Geometry: final body of the model. Coordinates: model frame, mm. Give positions to 0.01 mm unless a question says otherwise; leave off trailing zeros. Order: outer loops, then holes, each group sorted by start corner. A loop starts at its lowest first (then second) coordinate and runs counter-clockwise, first axis right, second up. Notation, with made-up numbers: (33.25, 43.25) -> (41.25, 43.25) arc R29 ccw to (41.25, 81.25) -> close; hole circle Ø4 at (74, 11). An arc over 180 degrees is marked (long way). Answer in a Markdown table with one row per item. Add a question column.
Q1. Contact query for flat-ended pins moving along their axis: P1, Ø0.7, axis at x = -114, z = 0.5, coming from the +Y side; P2, Ø0.7, axis at y = 174.5, z = 0.5, coming from the +X side. Output: stop coordinate, or through.
Q2. Cut plane C-C on y = 148.5. Return the cut outline in (x, z).
Q3. Cut plane B-B on x = -333.5. Return the cut outline in (y, z), and give its area (3 significant figures).
Q4. Cut plane A-A on z = 0.8. Return the cut outline in (x, y).
Q5. Line query: line 1 along Y through (x, z) = (-56, 0.35); line 2 along X through (y, z) = (202, 1.15). Output: solid intervals per line, ascending. Write a range as from..to.
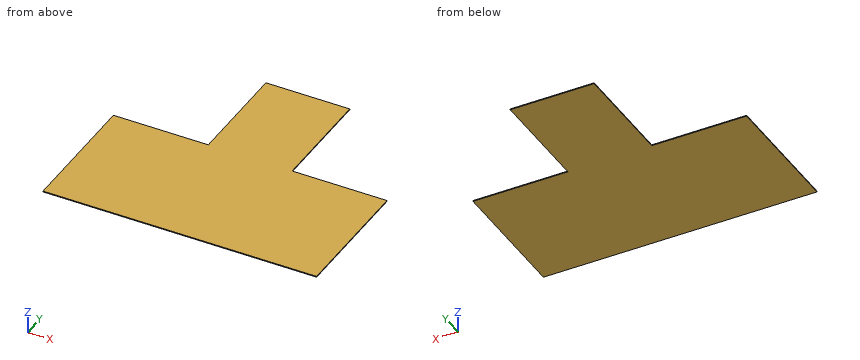
from build123d import *

# Parameters (mm, degrees)
F1_DEPTH = 1.4111111111
F2_DEPTH = 101.2317
F3_DEPTH = 66.675
F4_DEPTH = 66.675
F5_DEPTH = 47.498


# Not quite as in the source:
# - a length typed as a fraction of an inch, garbled in the dataset ("3 / 203.2 mm" for 3/8 in), is restored


with BuildPart() as f1:
    # F0 (on Top) → F1 (new body)
    with BuildSketch(Plane.XY):
        Polygon((-156.2699383586, 189.0532364881), (-290.5952983586, 189.0532364881), (-290.5952983586, -36.1571907997), (-375.8326183586, -36.1571907997), (-375.8326183586, -144.4919435119), (-71.0326183586, -144.4919435119), (-71.0326183586, -36.1571907997), (-156.2699383586, -36.1571907997), align=None)
    extrude(amount=F1_DEPTH)

    # F2 (add): faces of the model
    f2_faces = [f1.faces().sort_by_distance(p)[0] for p in [
        (-333.2139583586, -36.1571907997, 0.7055555556),
        (-113.6512783586, -36.1571907997, 0.7055555556),
    ]]
    extrude(f2_faces, amount=F2_DEPTH)

    # F3 (add): a face of the model
    f3_faces = [f1.faces().sort_by_distance(p)[0] for p in [
        (-71.0326183586, -39.7087171558, 0.7055555556),
    ]]
    extrude(f3_faces, amount=F3_DEPTH)

    # F4 (add): a face of the model
    f4_faces = [f1.faces().sort_by_distance(p)[0] for p in [
        (-375.8326183586, -39.7087171558, 0.7055555556),
    ]]
    extrude(f4_faces, amount=F4_DEPTH)

    # F5 (add): a face of the model
    f5_faces = [f1.faces().sort_by_distance(p)[0] for p in [
        (-223.4326183586, 189.0532364881, 0.7055555556),
    ]]
    extrude(f5_faces, amount=F5_DEPTH)


solid = f1.part
Completed:
| question | item | result |
|---|---|---|
| 1 | P1 | stops at y = 65.07 |
| 1 | P2 | stops at x = -156.27 |
| 2 | outline | (-290.6, 0) -> (-156.27, 0) -> (-156.27, 1.41) -> (-290.6, 1.41) -> close |
| 3 | outline | (-144.49, 0) -> (65.07, 0) -> (65.07, 1.41) -> (-144.49, 1.41) -> close |
| 3 | area | 296 mm² |
| 4 | outline | (-442.51, -144.49) -> (-4.36, -144.49) -> (-4.36, 65.07) -> (-156.27, 65.07) -> (-156.27, 236.55) -> (-290.6, 236.55) -> (-290.6, 65.07) -> (-442.51, 65.07) -> close |
| 5 | line 1 | y = -144.49..65.07 |
| 5 | line 2 | x = -290.6..-156.27 |
